Geometry check sheet. Reference: the model listing, model coordinates, mm. A direction names the side the tool comes from. Coordinates: 2 decimals unless noted, no trailing zeros. Write each loop counter-clockwise with the first axis right and the second up, starting at its lowest first coordinate (ties: lowest second). Pieces come first, ordered by that corner, then holes. Notation, with made-up numbers: (68.25, -35) - (92.25, -35) arc R14 cw to (92.25, -25) - close; hole circle Ø10 at (71.5, 74). An arc over 180 degrees is marked (long way). Answer as a JSON object with one key per item and string values. Group by question number.
from build123d import *

# Parameters (mm, degrees)
SKETCH_1_W          = 20
SKETCH_1_H          = 10
EXTRUDE_1_DEPTH     = 1.6
EXTRUDE_2_DEPTH     = 2
SKETCH_3_W          = 2
SKETCH_3_H          = 3.2
SKETCH_3_W_2        = 8.6
SKETCH_3_H_2        = 2
EXTRUDE_3_DEPTH     = 20
SKETCH_4_W          = 8.6
SKETCH_4_H          = 2
SKETCH_4_W_2        = 10
SKETCH_4_H_2        = 1.6
EXTRUDE_4_DEPTH     = 10
CUT_EXTRUDE_3_DEPTH = 15


with BuildPart() as part:
    # Эскиз1 → Бобышка-Вытянуть1 (new body)
    with BuildSketch(Plane(origin=(0, 0, 0), x_dir=(1, 0, 0), z_dir=(0, 1, 0))):
        with Locations((10, 5)):
            Rectangle(SKETCH_1_W, SKETCH_1_H)
    extrude(amount=EXTRUDE_1_DEPTH)

    # Эскиз2 → Бобышка-Вытянуть2 (add)
    with BuildSketch(Plane.ZY):
        Polygon((-14.5, 1.6), (4.5, 1.6), (4.5, -1.6), (-0.7, -1.6), (-0.7, -10.6), (-9.3, -10.6), (-9.3, -1.6), (-14.5, -1.6), align=None)
    extrude(amount=EXTRUDE_2_DEPTH)

    # Эскиз3 → Бобышка-Вытянуть3 (add)
    with BuildSketch(Plane(origin=(0, 0, 0), x_dir=(0, 0, -1), z_dir=(1, 0, 0))):
        with Locations((-3.5, 0)):
            Rectangle(SKETCH_3_W, SKETCH_3_H)
        with Locations((13.5, 0)):
            Rectangle(SKETCH_3_W, SKETCH_3_H)
        with Locations((5, -9.6)):
            Rectangle(SKETCH_3_W_2, SKETCH_3_H_2)
    extrude(amount=EXTRUDE_3_DEPTH)

    # Эскиз4 → Бобышка-Вытянуть4 (add)
    with BuildSketch(Plane(origin=(20, 0, 0), x_dir=(0, 0, -1), z_dir=(1, 0, 0))):
        with Locations((5, -9.6)):
            Rectangle(SKETCH_4_W, SKETCH_4_H)
        with Locations((5, 0.8)):
            Rectangle(SKETCH_4_W_2, SKETCH_4_H_2)
    extrude(amount=EXTRUDE_4_DEPTH)

    # Эскиз5 → Вырез-Вытянуть3 (cut)
    with BuildSketch(Plane.XZ.offset(10.6)):
        with BuildLine():
            Line((26.060660172, -6.060660172), (27.121320344, -5))
            Line((27.121320344, -5), (26.060660172, -3.939339828))
            ThreePointArc((26.060660172, -3.939339828), (23.5, -5), (26.060660172, -6.060660172))
        make_face()
    extrude(amount=-CUT_EXTRUDE_3_DEPTH, mode=Mode.SUBTRACT)


solid = part.part
(1) Section check D-D (x = 25). Record the cut outline in (y, z), and give its area (3 significant figures).
(2) Gauge pin test, flat ends, axial feed: pin 1 (1 mm diameter, centred on y = -0.5, z = 4, fed in from +X); pin 2 (4 mm diameter, centred on x = 16, y = -7, fed in from -Z); pin 3 (2.5 mm diameter, centred on x = 12, z = -12, fed in from -Y). Record the tip position at first contact, or that the pin passes through.
(3) Section check C-C (z = -1.5). Record the cut outline in (x, y), and give its area (3 significant figures).
(4) Draft check along Z on faces 6 (the face through (26.58, 0.79, -5.54)), 7 (the face through (9, 0, 4.5)), 8 (the face through (7, -1.6, -13)). Enter one of: +Z half, -Z half, draft (parallel to the pull), parting line (faces both ways), or undercut.
(5) Section check A-A (x = 12). Record the cut outline in (y, z).
(6) Set-up check for faces 1 (the face through (12, -9, -9.3)), 2 (the face through (26.58, -9.61, -5.54)), 3 (the face through (15, 0, -5)), 4 (the face through (15, -8.6, -5)), 5 (the face through (15, 1, -10)): record each of +Z, -Z, +X, -X, +Y, -Y from which the full face is reachable in a straight line by a thin tool's end or side.
(7) Section check B-B (y = -1.25). Record the cut outline in (x, z), and give its area (3 significant figures).
(8) Material ranges on L1, parallel to Y at x = 24, z = -1.5; L2, parallel to Z at x = 18, y = 1; L3, parallel to X at y = -6.25, z = -6.5, recorded low to high. Write a range as [from, to].
Conclusion:
{
 "1": {"outline": "(-10.6, -9.3) - (-8.6, -9.3) - (-8.6, -6.5) - (-10.6, -6.5) - close; (-10.6, -3.5) - (-8.6, -3.5) - (-8.6, -0.7) - (-10.6, -0.7) - close; (0, -10) - (1.6, -10) - (1.6, -6.5) - (0, -6.5) - close; (0, -3.5) - (1.6, -3.5) - (1.6, 0) - (0, 0) - close", "area": "22.4 mm^2"},
 "2": {"pin 1": "stops at x = 20", "pin 2": "stops at z = -9.3", "pin 3": "stops at y = -1.6"},
 "3": {"outline": "(-2, -10.6) - (30, -10.6) - (30, -8.6) - (0, -8.6) - (0, 0) - (30, 0) - (30, 1.6) - (-2, 1.6) - close", "area": "132 mm^2"},
 "4": {"face 6": "undercut", "face 7": "+Z half", "face 8": "draft"},
 "5": {"outline": "(-10.6, -9.3) - (-8.6, -9.3) - (-8.6, -0.7) - (-10.6, -0.7) - close; (-1.6, -14.5) - (1.6, -14.5) - (1.6, -12.5) - (-1.6, -12.5) - close; (-1.6, 2.5) - (1.6, 2.5) - (1.6, 4.5) - (-1.6, 4.5) - close; (0, -10) - (1.6, -10) - (1.6, 0) - (0, 0) - close"},
 "6": {"face 1": "-Z, +X, -X, -Y", "face 2": "+Y, -Y", "face 3": "+X", "face 4": "+Z, -Z, +X", "face 5": "+X, +Y, -Y"},
 "7": {"outline": "(-2, -14.5) - (20, -14.5) - (20, -12.5) - (0, -12.5) - (0, 2.5) - (20, 2.5) - (20, 4.5) - (-2, 4.5) - close", "area": "118 mm^2"},
 "8": {"L1": "y = [-10.6, -8.6], [0, 1.6]", "L2": "z = [-14.5, -12.5], [-10, 0], [2.5, 4.5]", "L3": "x = [-2, 0]"}
}
